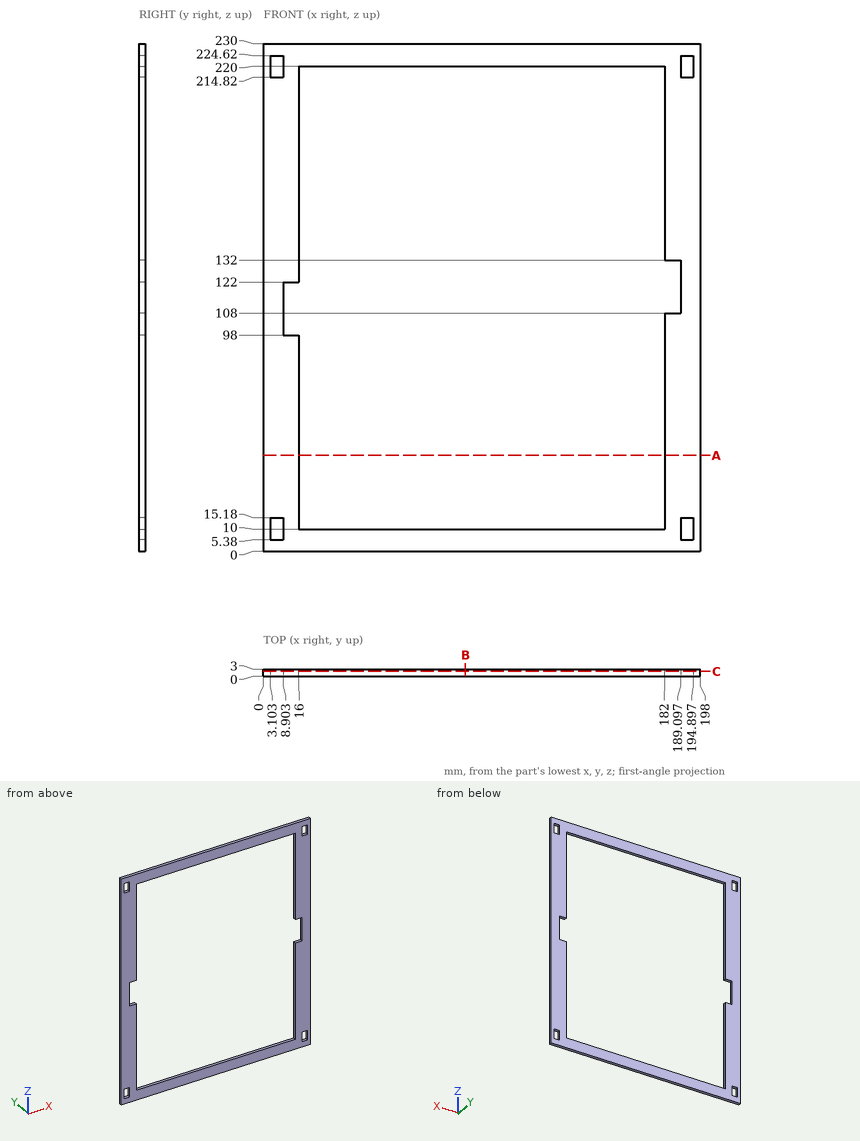
Answer from the drawing. Dimensions are ordinates in mm from the lowest x, y and z of the part. Round coordinates to 2 decimals unless told otherwise and drop trailing zeros. Write each loop counter-clockwise with the first axis right and the second up, starting at its lowest first coordinate (ties: lowest second). Pieces come first, ordered by that corner, then holes. Notation, with made-up numbers: M 61.5,-8.5 L 65.5,-8.5 A19 ccw 65.5,6.5 Z; hole C -22,58 d2. An arc over 180 degrees is marked long. Write each question's results on one line, items separated by ' | '. Start each with the question number.
Item 1: Find section A-A on z = 43.5. Write down the section's boundary in (x, y).
Item 2: Find section C-C on y = 2.15. Give the number of separate pieces and of enclosed holes in the cut face, and give its area (3 significant figures).
Item 3: Straight lines are drawn through the part: probe 1 along Z at (x, y) = (190, 0.1); probe 2 along X at (y, z) = (2.8, 16); probe 3 along Z at (x, y) = (17, 2.85). For each, find the intervals that lie inside material, in ascending order.
Item 4: Find section B-B on x = 91.5. Write down the section's boundary in (y, z), and give its area (3 significant figures).
Answer block:
1) outline: M 0,0 L 16,0 L 16,3 L 0,3 Z; M 182,0 L 198,0 L 198,3 L 182,3 Z
2) separate pieces: 1 | enclosed holes: 5 | area: 10,100 mm²
3) probe 1: z = 0 to 5.38, 15.18 to 214.82, 224.62 to 230 | probe 2: x = 0 to 16, 182 to 198 | probe 3: z = 0 to 10, 220 to 230
4) outline: M 0,0 L 3,0 L 3,10 L 0,10 Z; M 0,220 L 3,220 L 3,230 L 0,230 Z | area: 60.0 mm²
